Check sheet for the drawn part. Datum: minimum x, y, z corner. Units: mm. A direction names the side the tool comes from. Coordinates: 2 decimals unless noted, no trailing zeros. Loops run counter-clockwise (first coordinate to the right, second up) from the corner with the lowest first, then second, coordinate; pieces in that order, holes last. Notation, with made-up numbers: (34, -22) -> (40, -22) arc R32 ccw to (40, 13) -> close; hole circle Ø8 at (79, 40). An arc over 180 degrees is marked (long way). Use CSV: the item, a comma, the result in double quotes. Start each with the question number.
1. Sectioned sample at B-B, the plane y = 4. Record the cut outline in (x, z).
2. Thickness scan on L1, parallel to X at y = 4, z = 46.5; L2, parallel to Y at x = 2.75, z = 89; L3, parallel to Z at x = 9.5, y = 1.25. Record the ranges inside material, lowest first.
3. Set-up check for the marked faces 1, 2 and 3: record each of +Z, -Z, +X, -X, +Y, -Y from which the full face is reachable in a straight line by a thin tool's end or side.
4. Sectioned sample at C-C, the plane z = 32.5. Record the cut outline in (x, y), and give its area (3 significant figures).
5. Sectioned sample at A-A, the plane x = 10.5. Record the cut outline in (y, z) (1 decimal), and give its area (3 significant figures).
6. Gauge pin test, flat ends, axial feed: pin 1 (3 mm diameter, centred on x = 5.5, z = 12.5, fed in from +Y); pin 2 (0.8 mm diameter, centred on x = 8.5, y = 6, fed in from +Z); pin 3 (1 mm diameter, centred on y = 11, z = 94, fed in from +X); pin 4 (4 mm diameter, centred on y = 4, z = 73.5, fed in from +X). Record the tip position at first contact, or that the pin passes through.
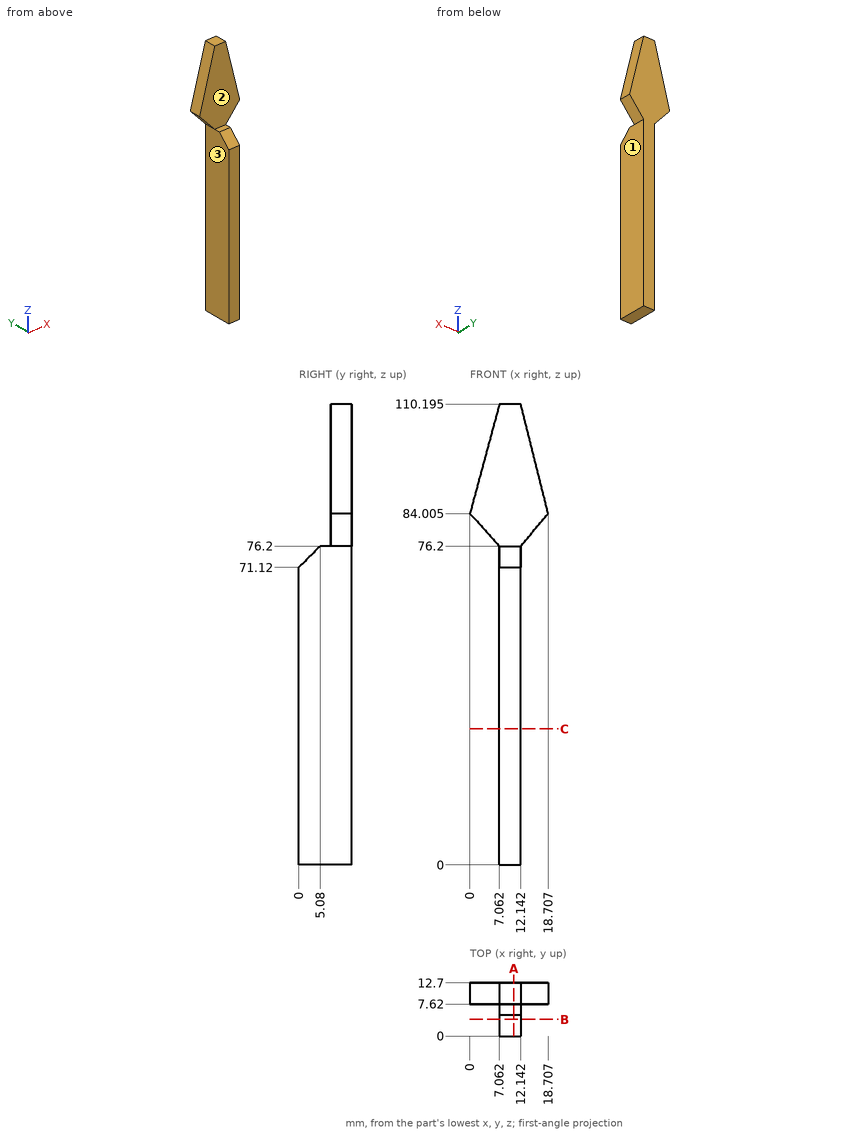
Completed:
1,outline,"(7.06, 0) -> (12.14, 0) -> (12.14, 75.12) -> (7.06, 75.12) -> close"
2,L1,"7.06 to 12.14"
2,L2,"7.62 to 12.7"
2,L3,"0 to 72.37"
3,face 1,"-Z, +X, +Y, -Y"
3,face 2,"+Z, +X, -X, -Y"
3,face 3,"-Z, -X, +Y, -Y"
4,outline,"(7.06, 0) -> (12.14, 0) -> (12.14, 12.7) -> (7.06, 12.7) -> close"
4,area,"64.5 mm²"
5,outline,"(0, 0) -> (12.7, 0) -> (12.7, 110.2) -> (7.6, 110.2) -> (7.6, 76.2) -> (5.1, 76.2) -> (0, 71.1) -> close"
5,area,"1,130 mm²"
6,pin 1,"through"
6,pin 2,"z = 76.2"
6,pin 3,"x = 16.33"
6,pin 4,"x = 12.14"
